```python
from build123d import *

# Parameters (mm, degrees)
EXTRUDE_1_DEPTH       = 330
EXTRUDE_3_DEPTH       = 330
PATTERN_CURVE_1_COUNT = 11
PATTERN_CURVE_1_PITCH = 10
SKETCH_3_R            = 2.25
CUT_EXTRUDE_1_DEPTH   = 6
SKETCH_4_R            = 1.6
SKETCH_4_R_2          = 2.1
SKETCH_4_R_3          = 2.5
SKETCH_4_R_4          = 1.1
CUT_EXTRUDE_2_DEPTH   = 6


with BuildPart() as part:
    # Эскиз1 → Вытянуть1 (new body)
    with BuildSketch(Plane.XY):
        with BuildLine():
            Line((0, 40), (1.528979332, 40))
            ThreePointArc((1.528979332, 40), (2.225614441, 39.717425624), (2.528547087, 39.029399052))
            Line((2.528547087, 39.029399052), (3.5, 6))
            Line((3.5, 6), (118.5, 6))
            Line((118.5, 6), (119.471452913, 39.029399052))
            ThreePointArc((119.471452913, 39.029399052), (119.774385559, 39.717425624), (120.471020668, 40))
            Line((120.471020668, 40), (122, 40))
            Line((122, 40), (122, 0))
            Line((122, 0), (0, 0))
            Line((0, 0), (0, 40))
        make_face()
    extrude(amount=EXTRUDE_1_DEPTH)

    # Эскиз2 → Вытянуть3 (add)
    with BuildSketch(Plane.XY.offset(330)):
        with BuildLine():
            Line((10.5, 39.5), (9.25, 6))
            Line((9.25, 6), (12.75, 6))
            Line((12.75, 6), (11.5, 39.5))
            ThreePointArc((11.5, 39.5), (11, 40), (10.5, 39.5))
        make_face()
    extrude_3 = extrude(amount=-EXTRUDE_3_DEPTH)

    # Кривая1: Вытянуть3 ×11
    with Locations(*[(i * PATTERN_CURVE_1_PITCH, 0, 0) for i in range(1, PATTERN_CURVE_1_COUNT)]):
        add(extrude_3)

    # Эскиз3 → Вырез-Вытянуть1 (cut)
    with BuildSketch(Plane.XZ):
        with Locations((26, 322)):
            Circle(SKETCH_3_R)
        with Locations((96, 322)):
            Circle(SKETCH_3_R)
        with Locations(Location((96, 8, 0), (0, 0, 180))):
            Circle(SKETCH_3_R)
        with Locations(Location((26, 8, 0), (0, 0, 180))):
            Circle(SKETCH_3_R)
    extrude(amount=-CUT_EXTRUDE_1_DEPTH, mode=Mode.SUBTRACT)

    # Эскиз4 → Вырез-Вытянуть2 (cut)
    with BuildSketch(Plane(origin=(1.487985642, 0, 27.400529356), x_dir=(1, 0, 0), z_dir=(0, -1, 0))):
        with Locations((65.512014358, 131.599470644)):
            Circle(SKETCH_4_R)
        with Locations((103.512014358, 188.999470644)):
            Circle(SKETCH_4_R)
        with Locations((60.512014358, 276.599470644)):
            Circle(SKETCH_4_R)
        with Locations((60.512014358, 141.599470644)):
            Circle(SKETCH_4_R)
        with Locations((65.512014358, -3.400529356)):
            Circle(SKETCH_4_R)
        with Locations((38.512014358, 113.599470644)):
            Circle(SKETCH_4_R_2)
        with Locations((109.632014358, 2.919470644)):
            Circle(SKETCH_4_R_3)
        with Locations((28.012014358, 76.099470644)):
            Circle(SKETCH_4_R)
        with Locations((48.712014358, 22.929470644)):
            Circle(SKETCH_4_R_4)
    extrude(amount=-CUT_EXTRUDE_2_DEPTH, mode=Mode.SUBTRACT)


solid = part.part
```
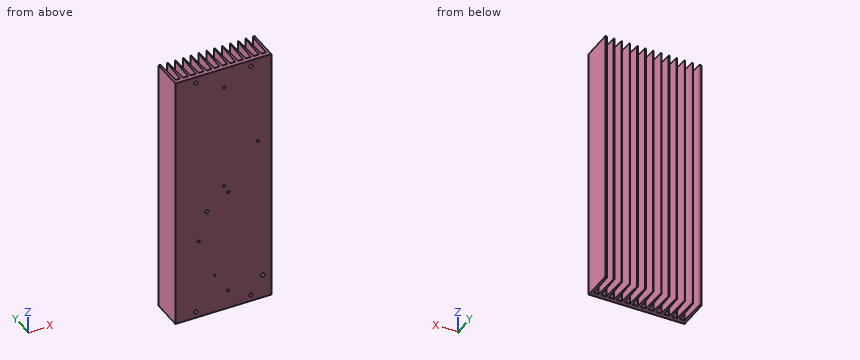
Input: part model. Units: mm. Frame: model coordinates. Coordinates: 2 decimals unless noted, no trailing zeros.
1) Pin query (flat end, axial travel): pin 1 Ø1.8 at (x, z) = (112, 29.5) entering from -Y; pin 2 Ø5 at (x, z) = (96, 105.5) entering from +Y. Return the tip coordinate at first contact, or that it passes through.
2) Section A-A on y = 17.5. State how many separate pieces and enclosed holes the cut face has, and give its area (3 significant figures).
3) Material intervals for line 1 along Z through (x, y) = (67, 1.4); line 2 along Z through (x, y) = (26, 2.8); line 3 along X through (y, z) = (2.7, 304), sorted ascending.
Check result:
1. pin 1: stops at y = 6
1. pin 2: stops at y = 6
2. separate pieces: 13
2. enclosed holes: 0
2. area: 11,700 mm2
3. line 1: z = 0 to 22.4, 25.6 to 157.4, 160.6 to 330
3. line 2: z = 0 to 5.75, 10.25 to 319.75, 324.25 to 330
3. line 3: x = 0 to 60.4, 63.6 to 122
